For this review, take the finished solid that the model builds, in its own axes (mm). Face numbers are marked on the shaded views. A direction names the side the tool comes from. Coordinates: 2 decimals unless noted, no trailing zeros. Write each loop counter-clockwise with the first axis right and the second up, starting at its lowest first coordinate (ties: lowest second). Pieces come first, ordered by that corner, then holes.
```python
from build123d import *

# Parameters (mm, degrees)
CUT_EXTRUDE1_REACH = 43
SKETCH2_R          = 10
CUT_EXTRUDE2_REACH = 28
SKETCH3_R          = 5.368889336
SKETCH3_4_R        = 5.368889336
CUT_EXTRUDE3_DEPTH = 11


with BuildPart() as part:
    # Sketch1 → Revolve1 (revolve)
    with BuildSketch(Plane(origin=(0, 0, 0), x_dir=(0, 0, -1), z_dir=(1, 0, 0))):
        Polygon((0, 0), (41, 0), (41, 16), (26, 18), (26, 35), (38, 38), (38, 48), (3, 48), (3, 38), (15, 35), (15, 18), (0, 16), align=None)
    revolve(axis=Axis((0, 0, 0), (0, 0, -1)))

    # Sketch2 → Cut-Extrude1 (cut, up to next)
    with BuildSketch(Plane.XY, mode=Mode.PRIVATE) as cut_extrude1_sk1:
        Circle(SKETCH2_R)
    cut_extrude1_tool1 = extrude(cut_extrude1_sk1.sketch, amount=-CUT_EXTRUDE1_REACH, mode=Mode.PRIVATE) & part.part
    add(cut_extrude1_tool1.solids().sort_by_distance((0, 0, 0))[0], mode=Mode.SUBTRACT)

    # Sketch3 → Cut-Extrude2 (cut, up to next)
    with BuildSketch(Plane.XY.offset(-15), mode=Mode.PRIVATE) as cut_extrude2_sk1:
        with Locations((0, 26.5)):
            Circle(SKETCH3_R)
    cut_extrude2_tool1 = extrude(cut_extrude2_sk1.sketch, amount=-CUT_EXTRUDE2_REACH, mode=Mode.PRIVATE) & part.part
    add(cut_extrude2_tool1.solids().sort_by_distance((0, 26.5, -15))[0], mode=Mode.SUBTRACT)

    # Sketch3<4> → Cut-Extrude3 (cut)
    with BuildSketch(Plane.XY.offset(-15)):
        with Locations((0, 26.5)):
            Circle(SKETCH3_4_R)
        with Locations((26.5, 0)):
            Circle(SKETCH3_4_R)
        with Locations((0, -26.5)):
            Circle(SKETCH3_4_R)
        with Locations((-26.5, 0)):
            Circle(SKETCH3_4_R)
    extrude(amount=-CUT_EXTRUDE3_DEPTH, mode=Mode.SUBTRACT)


solid = part.part
```
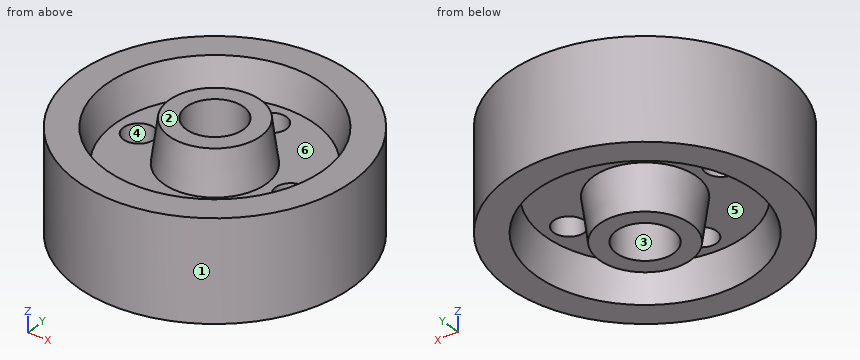
1) Consider section A-A (y = 0). Count the separate pieces of the cut face and the enclosed holes in it, then the cut area to 3 significant figures.
2) Clearance check with flat-ended pins moving along their axes: P1, Ø14, axis at x = -26.5, y = 0, coming from the +Z side; P2, Ø10, axis at x = -10.5, z = -30.5, coming from the -Y side; P3, Ø10, axis at y = 35.5, z = -23.5, coming from the +X side. State where each tip first meets the part, or that it passes through.
3) The part is to be moulded in two halves that separate along X. For the marked faces 1, 2 and 3, say which applies: pulls with the +X half, pulls with the -X half, needs draft (parallel to the pull), parting line crosses it, or undercut.
4) For L1, parallel to X at y = -10.5, z = -8; L2, parallel to Y at x = -7.5, z = -12; L3, parallel to Y at x = 10.5, z = -11, list the stretches that pass through material, from the lowest coordinate up.
5) Consider section C-C (z = -11). Give the boundary of the cut face in (x, y), then the cut area to 3 significant figures.
6) Tool access review of the marked faces 4, 5 and 6: name each direction out of +Z, -Z, +X, -X, +Y, -Y from which nothing blocks a thin tool from reaching the whole face with its end or side.
Results:
1. separate pieces: 4
1. enclosed holes: 0
1. area: 1,570 mm2
2. P1: stops at z = -15
2. P2: stops at y = -47.68
2. P3: stops at x = 37.06
3. face 1: parting line crosses it
3. face 2: needs draft
3. face 3: undercut
4. L1: x = -46.84 to -35.22, -13.45 to 13.45, 35.22 to 46.84
4. L2: y = -47.41 to -34.95, -15.92 to -6.61, 6.61 to 15.92, 34.95 to 47.41
4. L3: y = -46.84 to -34.43, -13.96 to 13.96, 34.43 to 46.84
5. outline: circle Ø96 at (0, 0); circle Ø34.93 at (0, 0); hole circle Ø72 at (0, 0); hole circle Ø20 at (0, 0)
5. area: 3,810 mm2
6. face 4: +Z, -Z
6. face 5: -Z
6. face 6: +Z
